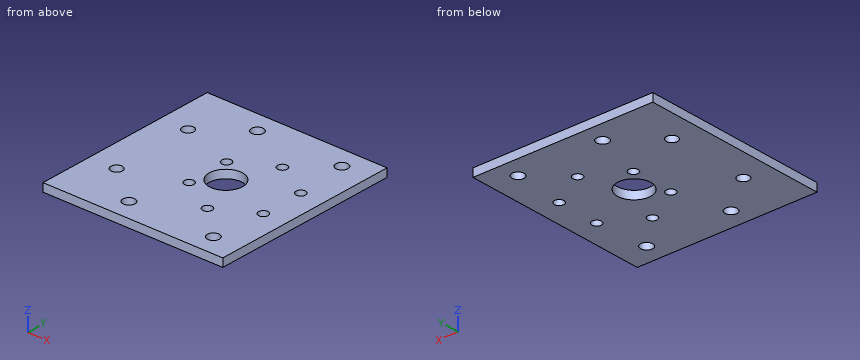
from build123d import *

# Parameters (mm, degrees)
SKETCH_1_W          = 40
SKETCH_1_H          = 29
EXTRUDE_1_DEPTH     = 3
SKETCH_3_W          = 40
SKETCH_3_H          = 3
EXTRUDE_2_DEPTH     = 10
SKETCH_4_W          = 40
SKETCH_4_H          = 3
EXTRUDE_3_DEPTH     = 10
SKETCH_6_W          = 3
SKETCH_6_H          = 49
EXTRUDE_5_DEPTH     = 42
SKETCH_8_W          = 3
SKETCH_8_H          = 49
EXTRUDE_6_DEPTH     = 2
SKETCH_9_W          = 3
SKETCH_9_H          = 49
EXTRUDE_7_DEPTH     = 2
SKETCH_10_W         = 86
SKETCH_10_H         = 3
EXTRUDE_8_DEPTH     = 10
SKETCH_11_W         = 86
SKETCH_11_H         = 3
EXTRUDE_9_DEPTH     = 10
SKETCH_12_R         = 2.2
CUT_EXTRUDE_3_DEPTH = 7.5
SKETCH_7_R          = 1.75
SKETCH_7_R_2        = 6.1
CUT_EXTRUDE_4_DEPTH = 10
SKETCH_13_R         = 2.1
CUT_EXTRUDE_5_DEPTH = 10
SKETCH_14_W         = 3
SKETCH_14_H         = 69
CUT_EXTRUDE_6_DEPTH = 20


with BuildPart() as part:
    # Sketch 1 → Extrude 1 (new body)
    with BuildSketch(Plane.XY):
        Rectangle(SKETCH_1_W, SKETCH_1_H)
    extrude(amount=EXTRUDE_1_DEPTH)

    # Sketch 3 → Extrude 2 (add)
    with BuildSketch(Plane.XZ.offset(14.5)):
        with Locations((0, 1.5)):
            Rectangle(SKETCH_3_W, SKETCH_3_H)
    extrude(amount=EXTRUDE_2_DEPTH)

    # Sketch 4 → Extrude 3 (add)
    with BuildSketch(Plane(origin=(0, 14.5, 0), x_dir=(1, 0, 0), z_dir=(0, 1, 0))):
        with Locations((0, -1.5)):
            Rectangle(SKETCH_4_W, SKETCH_4_H)
    extrude(amount=EXTRUDE_3_DEPTH)

    # Sketch 6 → Extrude 5 (add)
    with BuildSketch(Plane(origin=(20, 0, 0), x_dir=(0, 0, -1), z_dir=(1, 0, 0))):
        with Locations((-1.5, 0)):
            Rectangle(SKETCH_6_W, SKETCH_6_H)
    extrude(amount=EXTRUDE_5_DEPTH)

    # Sketch 8 → Extrude 6 (add)
    with BuildSketch(Plane.ZY.offset(20)):
        with Locations((1.5, 0)):
            Rectangle(SKETCH_8_W, SKETCH_8_H)
    extrude(amount=EXTRUDE_6_DEPTH)

    # Sketch 9 → Extrude 7 (add)
    with BuildSketch(Plane(origin=(62, 0, 0), x_dir=(0, 0, -1), z_dir=(1, 0, 0))):
        with Locations((-1.5, 0)):
            Rectangle(SKETCH_9_W, SKETCH_9_H)
    extrude(amount=EXTRUDE_7_DEPTH)

    # Sketch 10 → Extrude 8 (add)
    with BuildSketch(Plane.XZ.offset(24.5)):
        with Locations((21, 1.5)):
            Rectangle(SKETCH_10_W, SKETCH_10_H)
    extrude(amount=EXTRUDE_8_DEPTH)

    # Sketch 11 → Extrude 9 (add)
    with BuildSketch(Plane(origin=(0, 24.5, 0), x_dir=(1, 0, 0), z_dir=(0, 1, 0))):
        with Locations((21, -1.5)):
            Rectangle(SKETCH_11_W, SKETCH_11_H)
    extrude(amount=EXTRUDE_9_DEPTH)

    # Sketch 12 → Cut-Extrude 3 (cut)
    with BuildSketch(Plane.XY.offset(3)):
        with Locations((34, -27)):
            Circle(SKETCH_12_R)
        with Locations((34, 27)):
            Circle(SKETCH_12_R)
        with Locations((3, -27)):
            Circle(SKETCH_12_R)
        with Locations((3, 27)):
            Circle(SKETCH_12_R)
    extrude(amount=-CUT_EXTRUDE_3_DEPTH, mode=Mode.SUBTRACT)

    # Sketch 7 → Cut-Extrude 4 (cut)
    with BuildSketch(Plane.XY.offset(3)):
        with Locations((35.63990011, 7.875)):
            Circle(SKETCH_7_R)
        with Locations((35.63990011, -7.875)):
            Circle(SKETCH_7_R)
        with Locations((15, 0)):
            Circle(SKETCH_7_R_2)
        with Locations((22, 15.75)):
            Circle(SKETCH_7_R)
        with Locations((22, -15.75)):
            Circle(SKETCH_7_R)
        with Locations((8.36009989, 7.875)):
            Circle(SKETCH_7_R)
        with Locations((8.36009989, -7.875)):
            Circle(SKETCH_7_R)
    extrude(amount=-CUT_EXTRUDE_4_DEPTH, mode=Mode.SUBTRACT)

    # Sketch 13 → Cut-Extrude 5 (cut)
    with BuildSketch(Plane.XY.offset(3)):
        with Locations((-12, -15)):
            Circle(SKETCH_13_R)
        with Locations((-12, 15)):
            Circle(SKETCH_13_R)
    extrude(amount=-CUT_EXTRUDE_5_DEPTH, mode=Mode.SUBTRACT)

    # Sketch 14 → Cut-Extrude 6 (cut)
    with BuildSketch(Plane(origin=(64, 0, 0), x_dir=(0, 0, -1), z_dir=(1, 0, 0))):
        with Locations((-1.5, 0)):
            Rectangle(SKETCH_14_W, SKETCH_14_H)
    extrude(amount=-CUT_EXTRUDE_6_DEPTH, mode=Mode.SUBTRACT)


solid = part.part
Could you check a few things on this model? Use its own coordinates, in mm. Round coordinates to 2 decimals unless told otherwise and drop trailing zeros. Order: outer loops, then holes, each group sorted by start corner. A loop starts at its lowest first (then second) coordinate and runs counter-clockwise, first axis right, second up.
Q1. Imagine slicing it at C-C, the plane y = 27. List the corners of the cut face in (x, z) for me, then the cut area to 3 significant figures.
Geometry says:
outline: (-22, 0) - (0.8, 0) - (0.8, 3) - (-22, 3) - close; (5.2, 0) - (31.8, 0) - (31.8, 3) - (5.2, 3) - close; (36.2, 0) - (44, 0) - (44, 3) - (36.2, 3) - close
area: 172 mm2
Q2. Imagine slicing it at A-A, the plane x = 15. List the corners of the cut face in (y, z) for me.
Geometry says:
outline: (-34.5, 0) - (-6.1, 0) - (-6.1, 3) - (-34.5, 3) - close; (6.1, 0) - (34.5, 0) - (34.5, 3) - (6.1, 3) - close
Q3. Please list where these lines run through material, in increasing order: probe 1 along Y at (x, z) = (-12, 1.35); probe 2 along Y at (x, z) = (23, 0.4); probe 3 along Y at (x, z) = (9.5, 0.25).
Geometry says:
probe 1: y = -34.5 to -17.1, -12.9 to 12.9, 17.1 to 34.5
probe 2: y = -34.5 to -17.19, -14.31 to 14.31, 17.19 to 34.5
probe 3: y = -34.5 to -9.2, -6.55 to -2.64, 2.64 to 6.55, 9.2 to 34.5
Q4. Imagine slicing it at B-B, the plane x = 22. List the corners of the cut face in (y, z) for me, then the cut area to 3 significant figures.
Geometry says:
outline: (-34.5, 0) - (-17.5, 0) - (-17.5, 3) - (-34.5, 3) - close; (-14, 0) - (14, 0) - (14, 3) - (-14, 3) - close; (17.5, 0) - (34.5, 0) - (34.5, 3) - (17.5, 3) - close
area: 186 mm2
Q5. I'm going to push a flat-ended pin straight in: P1, Ø7.5, axis at x = 15, y = 0, coming from the -Z side. Where does the tip first touch, or does it pass through?
Geometry says:
P1: passes through
Q6. Imagine slicing it at D-D, the plane z = 1.2. State how many separate pieces and enclosed holes the cut face has, then the cut area to 3 significant figures.
Geometry says:
separate pieces: 1
enclosed holes: 13
area: 4,290 mm2
